The model under review builds one solid part; all positions refer to its coordinate system, in mm. Face numbers are marked on the shaded views. A direction names the side the tool comes from. Give positions to 0.01 mm unless a question says otherwise; leave off trailing zeros. Loops run counter-clockwise (first coordinate to the right, second up) from the corner with the lowest first, then second, coordinate; pieces in that order, holes last. Notation, with made-up numbers: (-12, 53.25) - (46, 53.25) arc R28 cw to (46, 71.25) - close; hole circle Ø3 at (6, -29.5). An arc over 180 degrees is marked (long way). Answer as a JSON object with one key per item and string values.
from build123d import *

# Parameters (mm, degrees)
SKETCH1_W           = 40.64
SKETCH1_H           = 40.3352
BOSS_EXTRUDE1_DEPTH = 20.4724
SKETCH3_R           = 2.921
SKETCH3_R_2         = 0.6985
BOSS_EXTRUDE2_DEPTH = 5.08
SKETCH4_R           = 1
CUT_EXTRUDE1_DEPTH  = 61.808363905


with BuildPart() as part:
    # Sketch1 → Boss-Extrude1 (new body)
    with BuildSketch(Plane(origin=(0, 0, 0), x_dir=(1, 0, 0), z_dir=(0, 1, 0))):
        with Locations((20.32, 20.1676)):
            Rectangle(SKETCH1_W, SKETCH1_H)
    extrude(amount=BOSS_EXTRUDE1_DEPTH)

    # Sketch3 → Boss-Extrude2 (add)
    with BuildSketch(Plane.ZY):
        with Locations(Location((-10.541, 10.2362, 0), (0, 0, 180))):
            Circle(SKETCH3_R)
        with Locations((-10.541, 10.2362)):
            Circle(SKETCH3_R_2, mode=Mode.SUBTRACT)
    extrude(amount=BOSS_EXTRUDE2_DEPTH)

    # Sketch4 → Cut-Extrude1 (cut, through all)
    with BuildSketch(Plane.ZY):
        with Locations((-37.8352, 17.736)):
            Circle(SKETCH4_R)
        with Locations((-37.8352, 2.736)):
            Circle(SKETCH4_R)
        with Locations((-22.8352, 17.736)):
            Circle(SKETCH4_R)
        with Locations((-22.8352, 2.736)):
            Circle(SKETCH4_R)
    extrude(amount=-CUT_EXTRUDE1_DEPTH, mode=Mode.SUBTRACT)


solid = part.part
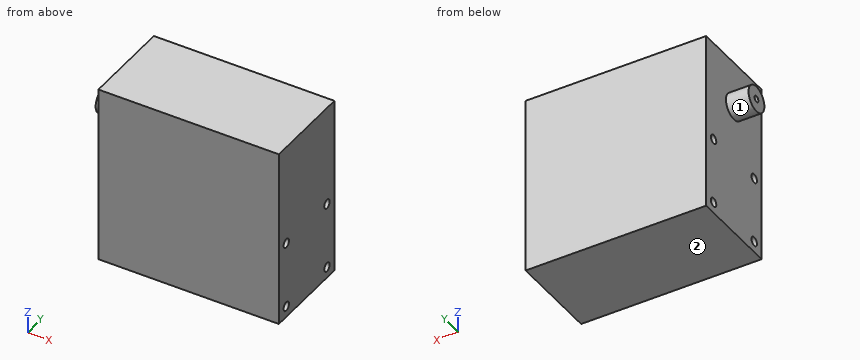
Q1. Clearance check with flat-ended pins moving along their axes: pin 1 Ø0.7 at (y, z) = (10, -10.5) entering from -X; pin 2 Ø1.8 at (y, z) = (17.74, -22.84) entering from +X. State where each tip first meets the part, or that it passes through.
Results:
{"pin 1": "stops at x = 0", "pin 2": "passes through"}
Q2. Consider section C-C, the plane y = 4.5. State the section outline as (x, z) points, plus the area to 3 significant figures.
Results:
{"outline": "(0, -40.34) - (40.64, -40.34) - (40.64, 0) - (0, 0) - close", "area": "1,640 mm^2"}
Q3. For the marked faces 1 and 2, list the 3-axis set-ups (+Z, -Z, +X, -X, +Y, -Y) from which the entire face can be reached by the end or side of a thin tool; tool diameter is ignored.
Results:
{"face 1": "-X", "face 2": "-Z, +X, -X, +Y, -Y"}
Q4. To check wall thickness, follow probe 1 along Y at (x, z) = (3, -23); probe 2 along Z at (x, y) = (6.5, 17); probe 3 along Z at (x, y) = (10, 3). State the ranges of each line that lie inside material, in increasing order. Write a range as [from, to].
Results:
{"probe 1": "y = [0, 1.75], [3.72, 16.75], [18.72, 20.47]", "probe 2": "z = [-40.34, -38.51], [-37.16, -23.51], [-22.16, 0]", "probe 3": "z = [-40.34, -38.8], [-36.87, -23.8], [-21.87, 0]"}
Q5. Consider section D-D, the plane z = -5. State the section outline as (x, y) points, plus the area to 3 significant figures.
Results:
{"outline": "(0, 0) - (40.64, 0) - (40.64, 20.47) - (0, 20.47) - close", "area": "832 mm^2"}
Q6. Consider section A-A, the plane x = 31.5. State the section outline as (y, z) points.
Results:
{"outline": "(0, -40.34) - (20.47, -40.34) - (20.47, 0) - (0, 0) - close; hole circle Ø2 at (2.74, -37.84); hole circle Ø2 at (2.74, -22.84); hole circle Ø2 at (17.74, -37.84); hole circle Ø2 at (17.74, -22.84)"}
Q7. Consider section B-B, the plane z = -37.5. State the section outline as (x, y) points, plus the area to 3 significant figures.
Results:
{"outline": "(0, 0) - (40.64, 0) - (40.64, 1.79) - (0, 1.79) - close; (0, 3.68) - (40.64, 3.68) - (40.64, 16.79) - (0, 16.79) - close; (0, 18.68) - (40.64, 18.68) - (40.64, 20.47) - (0, 20.47) - close", "area": "679 mm^2"}
